```python
from build123d import *

# Parameters (mm, degrees)
F0_W     = 609.6
F0_H     = 609.6
F1_DEPTH = 101.6
F2_W     = 101.6
F2_H     = 152.4
F3_DEPTH = 101.6
F4_R     = 12.7
F5_DEPTH = 609.6
F6_W     = 114.3
F6_H     = 609.6
F7_DEPTH = 76.2
F8_R     = 12.7
F9_DEPTH = 114.3


with BuildPart() as f1:
    # F0 (on Top) → F1 (new body)
    with BuildSketch(Plane.XY):
        with Locations((178.062361, 224.069413)):
            Rectangle(F0_W, F0_H)
    extrude(amount=F1_DEPTH)

    # F2 (on Top) → F3 (cut)
    with BuildSketch(Plane.XY):
        with Locations((393.962361, -4.530587)):
            Rectangle(F2_W, F2_H)
        with Locations((-37.837639, -4.530587)):
            Rectangle(F2_W, F2_H)
        with Locations((-37.837639, 452.669413)):
            Rectangle(F2_W, F2_H)
        with Locations((393.962361, 452.669413)):
            Rectangle(F2_W, F2_H)
    extrude(amount=F3_DEPTH, mode=Mode.SUBTRACT)

    # F4 (on face) → F5 (join)
    with BuildSketch(Plane(origin=(-126.737639, 0, 0), x_dir=(0, -1, 0), z_dir=(-1, 0, 0))):
        with Locations((-452.669413, 50.8)):
            Circle(F4_R)
        with Locations((4.530587, 50.8)):
            Circle(F4_R)
    extrude(amount=-F5_DEPTH)

    # F6 (on face) → F7 (cut)
    with BuildSketch(Plane.XY.offset(101.6)):
        with Locations((178.062361, 224.069413)):
            Rectangle(F6_W, F6_H)
    extrude(amount=-F7_DEPTH, mode=Mode.SUBTRACT)

    # F8 (on face) → F9 (join, through all)
    with BuildSketch(Plane.YZ.offset(120.912361)):
        with Locations((20.869413, 76.2)):
            Circle(F8_R)
        with Locations((325.669413, 76.2)):
            Circle(F8_R)
    extrude(amount=F9_DEPTH)


solid = f1.part
```
Geometry check sheet. Reference: the model listing, model coordinates, mm. A direction names the side the tool comes from. Give positions to 0.01 mm unless a question says otherwise; leave off trailing zeros. Order: outer loops, then holes, each group sorted by start corner. A loop starts at its lowest first (then second) coordinate and runs counter-clockwise, first axis right, second up. Notation, with made-up numbers: (54.5, 30.25) - (63.5, 30.25) arc R35 cw to (63.5, 63.25) - close; hole circle Ø1 at (-7.5, -36.75). An arc over 180 degrees is marked (long way). Answer in a Markdown table with one row per item. Add a question column.
Q1. Mould release check, pull along X, two halves, no side actions. Record for faces 1 (the flat face through (-108, 528.869, 50)), 2 (the flat face through (393, 376.469, 50)), 3 (the flat face through (-126.738, 228, 52)): pulls with the +X half, pulls with the -X half, needs draft (parallel to the pull), parting line crosses it, or undercut.
Q2. Cross-section at B-B, the plane y = 21. Enter the section's corners in (x, z), then the cut area to 3 significant figures.
Q3. Material ranges on probe 1 along X at (y, z) = (47, 69.5); probe 2 along Y at (x, z) = (-21.5, 49.5); probe 3 along Y at (x, z) = (351, 52.5), recorded low to high. Write a range as from..to.
Q4. Cross-section at D-D, the plane z = 7. Enter the section's corners in (x, y), then the cut area to 3 significant figures.
Q5. Cross-section at C-C, the plane x = 142. Enter the section's corners in (y, z), then the cut area to 3 significant figures.
Q6. Gauge pin test, flat ends, axial feed: pin 1 (4 mm diameter, centred on x = 162, z = 67, fed in from -Y); pin 2 (10 mm diameter, centred on x = 147.5, z = 62.5, fed in from +Y); pin 3 (5 mm diameter, centred on x = 368, z = 84.5, fed in from -Y). Record the tip position at first contact, or that the pin passes through.
Q7. Tool access check on faces 4 (the flat face through (393, 71.669, 50)), 5 (the cylindrical face through (393.251, 462.748, 43.072)), 6 (the flat face through (176, -80.731, 16)). Record the directions out of +Z, -Z, +X, -X, +Y, -Y that give a thin tool (end or side, any length) a straight path to the whole face; none if there is none.
Check values:
| question | item | result |
|---|---|---|
| 1 | face 1 | needs draft |
| 1 | face 2 | undercut |
| 1 | face 3 | pulls with the -X half |
| 2 | outline | (-126.74, 0) - (-88.64, 0) - (-88.64, 101.6) - (-126.74, 101.6) - close; (12.96, 0) - (343.16, 0) - (343.16, 101.6) - (235.21, 101.6) - (235.21, 88.9) - (120.91, 88.9) - (120.91, 101.6) - (12.96, 101.6) - close; (444.76, 0) - (482.86, 0) - (482.86, 101.6) - (444.76, 101.6) - close; hole (120.91, 25.4) - (235.21, 25.4) - (235.21, 63.5) - (120.91, 63.5) - close |
| 2 | area | 35,500 mm^2 |
| 3 | probe 1 | x = -126.74..-88.64, 12.96..120.91, 235.21..343.16, 444.76..482.86 |
| 3 | probe 2 | y = -17.16..8.1, 71.67..376.47, 440.04..465.3 |
| 3 | probe 3 | y = -17.12..8.06, 71.67..376.47, 440.08..465.26 |
| 4 | outline | (-126.74, -80.73) - (-88.64, -80.73) - (-88.64, 71.67) - (12.96, 71.67) - (12.96, -80.73) - (343.16, -80.73) - (343.16, 71.67) - (444.76, 71.67) - (444.76, -80.73) - (482.86, -80.73) - (482.86, 528.87) - (444.76, 528.87) - (444.76, 376.47) - (343.16, 376.47) - (343.16, 528.87) - (12.96, 528.87) - (12.96, 376.47) - (-88.64, 376.47) - (-88.64, 528.87) - (-126.74, 528.87) - close |
| 4 | area | 310,000 mm^2 |
| 5 | outline | (-80.73, 0) - (528.87, 0) - (528.87, 25.4) - (-80.73, 25.4) - close; circle Ø25.4 at (20.87, 76.2); circle Ø25.4 at (325.67, 76.2) |
| 5 | area | 16,500 mm^2 |
| 6 | pin 1 | stops at y = 10.41 |
| 6 | pin 2 | stops at y = 334.92 |
| 6 | pin 3 | stops at y = 71.67 |
| 7 | face 4 | +Z, -Z |
| 7 | face 5 | none |
| 7 | face 6 | +Z, -Z, +X, -X, -Y |
